```python
from build123d import *

# Parameters (mm, degrees)
F1_DEPTH = 63.5
F3_DEPTH = 31.75


with BuildPart() as f1:
    # F0 (on Front) → F1 (new body, symmetric)
    with BuildSketch(Plane.XZ):
        with BuildLine():
            ThreePointArc((63.5, 0), (18.598719, 18.598719), (0, 63.5))
            Line((0, 63.5), (-63.5, 63.5))
            Line((-63.5, 63.5), (-63.5, -63.5))
            Line((-63.5, -63.5), (63.5, -63.5))
            Line((63.5, -63.5), (63.5, 0))
        make_face()
    extrude(amount=F1_DEPTH, both=True)

    # F2 (on Front) → F3 (join, symmetric)
    with BuildSketch(Plane.XZ):
        with BuildLine():
            Line((0, 127), (0, 0))
            Line((0, 0), (127, 0))
            Line((127, 0), (127, 63.5))
            ThreePointArc((127, 63.5), (82.098719, 82.098719), (63.5, 127))
            Line((63.5, 127), (0, 127))
        make_face()
    extrude(amount=F3_DEPTH, both=True)


solid = f1.part
```
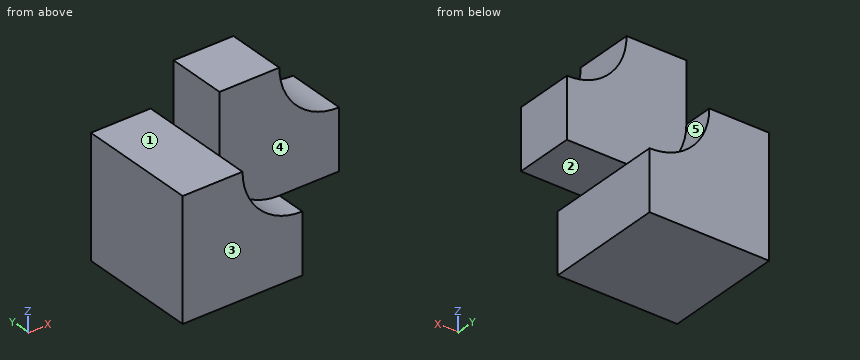
Design review of the part built by this model. Coordinates are the model's own, in mm. Face numbers are marked on the shaded views. A direction names the side the tool comes from. Round coordinates to 2 decimals unless told otherwise and drop trailing zeros. Order: outer loops, then holes, each group sorted by start corner. A loop starts at its lowest first (then second) coordinate and runs counter-clockwise, first axis right, second up. Notation, with made-up numbers: (80.25, 27.25) - (86.25, 27.25) arc R19 ccw to (86.25, 49.25) - close; hole circle Ø2 at (4.5, 11.5). An arc over 180 degrees is marked (long way). Return JSON: item names as keys, results as strings.
Q1. Wall thickness on L1, parallel to Y at x = 1.5, z = 83.5; L2, parallel to Z at x = -16, y = -14: over which ranges is each line inside the solid? List them lowest first. Write a range as [from, to].
Computed values:
{"L1": "y = [-31.75, 31.75]", "L2": "z = [-63.5, 63.5]"}
Q2. Consider section B-B on z = 6. Write out the cut boundary in (x, y), plus the area to 3 significant figures.
Computed values:
{"outline": "(-63.5, -63.5) - (36.56, -63.5) - (36.56, -31.75) - (127, -31.75) - (127, 31.75) - (36.56, 31.75) - (36.56, 63.5) - (-63.5, 63.5) - close", "area": "18,500 mm2"}
Q3. For pin 1 Ø12 at (x, z) = (71.5, 18.5) entering from +Y; pin 2 Ø19 at (x, y) = (-18.5, -7) entering from +Z; pin 3 Ø19 at (x, y) = (86.5, 2) entering from -Z, all flat-tipped, find the tip position at first contact; note any pin that passes through.
Computed values:
{"pin 1": "stops at y = 31.75", "pin 2": "stops at z = 63.5", "pin 3": "stops at z = 0"}
Q4. Consider section C-C on y = 7. Write out the cut boundary in (x, z).
Computed values:
{"outline": "(-63.5, -63.5) - (63.5, -63.5) - (63.5, 0) - (127, 0) - (127, 63.5) arc R63.5 cw to (63.5, 127) - (0, 127) - (0, 63.5) - (-63.5, 63.5) - close"}
Q5. Consider section D-D on x = 76.5. Write out the cut boundary in (y, z).
Computed values:
{"outline": "(-31.75, 0) - (31.75, 0) - (31.75, 88.5) - (-31.75, 88.5) - close"}
Q6. Consider section A-A on y = 40. Write out the cut boundary in (x, z).
Computed values:
{"outline": "(-63.5, -63.5) - (63.5, -63.5) - (63.5, 0) arc R63.5 cw to (0, 63.5) - (-63.5, 63.5) - close"}
Q7. Machinability: for the marked faces 1, 2, 3, 4 and 5, which of the approach directions +Z, -Z, +X, -X, +Y, -Y give a long, thin tool a straight path to every point of the face, cutting with its end or side? Answer none if there is none.
Computed values:
{"face 1": "+Z, -X, +Y, -Y", "face 2": "-Z, +X, +Y, -Y", "face 3": "+Z, -Z, +X, -X, -Y", "face 4": "+Z, +X, -Y", "face 5": "+Z, +X, +Y"}
